```python
from build123d import *

# Parameters (mm, degrees)
SKETCH3_R               = 0.75
CUT_EXTRUDE1_DEPTH      = 1.009552721
CUT_EXTRUDE1_DEPTH_BACK = 5
SKETCH5_R               = 0.830043706
CUT_EXTRUDE3_DEPTH      = 5
SKETCH6_W               = 0.475158235
SKETCH6_H               = 2.253950387
SKETCH6_W_2             = 0.475158234
CUT_EXTRUDE4_DEPTH      = 10
CUT_EXTRUDE4_DEPTH_BACK = 10


with BuildPart() as part:
    # Sketch1 → Revolve1 (revolve)
    with BuildSketch(Plane.XY):
        with BuildLine():
            Line((0, 0), (1, 0))
            Line((1, 0), (1, -12))
            Line((1, -12), (1, -12.602750297))
            add(Edge.make_bspline(
                [(1, -12.602750297), (0.79843866, -14.189468734), (4.052548494, -14.158592974), (3.356440043, -16.677675858), (3.45632985, -17.31657115)],
                knots=[0, 0, 0, 0, 0.610593848, 1, 1, 1, 1], degree=3))
            Line((3.45632985, -17.31657115), (3.084044258, -17.31657115))
            add(Edge.make_bspline(
                [(0, -12.602750297), (-0.217127131, -15.249179965), (3.341761348, -14.727809166), (3.084044258, -17.31657115)],
                knots=[0, 0, 0, 0, 1, 1, 1, 1], degree=3))
            add(Edge.make_bspline(
                [(0, -12), (0, -12.602750297)],
                knots=[0, 0, 1, 1], degree=1))
            Line((0, -12), (0, 0))
        make_face()
    revolve(axis=Axis((3.879111396, 0, 0), (0, -1, 0)))

    # Sketch3 → Cut-Extrude1 (cut, two sides)
    with BuildSketch(Plane(origin=(7.7582228, 0, 0), x_dir=(0, 0, -1), z_dir=(1, 0, 0))) as cut_extrude1_sk:
        with Locations((0, -1.4)):
            Circle(SKETCH3_R)
    extrude(amount=CUT_EXTRUDE1_DEPTH, mode=Mode.SUBTRACT)
    extrude(cut_extrude1_sk.sketch, amount=-CUT_EXTRUDE1_DEPTH_BACK, mode=Mode.SUBTRACT)

    # Sketch5 → Cut-Extrude3 (cut)
    with BuildSketch(Plane(origin=(-0.0208886, 0, 0), x_dir=(0, 0, -1), z_dir=(1, 0, 0))):
        with Locations((0, -1.4)):
            Circle(SKETCH5_R)
    extrude(amount=CUT_EXTRUDE3_DEPTH, mode=Mode.SUBTRACT)

    # Sketch6 → Cut-Extrude4 (cut, two sides)
    with BuildSketch(Plane.XY) as cut_extrude4_sk:
        with Locations((0.237579118, -1.525266711)):
            Rectangle(SKETCH6_W, SKETCH6_H)
        with Locations((7.520643674, -1.525266711)):
            Rectangle(SKETCH6_W_2, SKETCH6_H)
    extrude(amount=CUT_EXTRUDE4_DEPTH, mode=Mode.SUBTRACT)
    extrude(cut_extrude4_sk.sketch, amount=-CUT_EXTRUDE4_DEPTH_BACK, mode=Mode.SUBTRACT)


solid = part.part
```
The listing builds one solid part. Answer for the finished solid, in the listing's coordinates (mm). A direction names the side the tool comes from. Give positions to 0.01 mm unless a question says otherwise; leave off trailing zeros. Order: outer loops, then holes, each group sorted by start corner. A loop starts at its lowest first (then second) coordinate and runs counter-clockwise, first axis right, second up. Notation, with made-up numbers: (-14, 61) - (15, 61) arc R25 ccw to (15, 78) - close; hole circle Ø10 at (-36.5, 13). An arc over 180 degrees is marked (long way). Use one line per item in the form item = value. Start each with the question number.
(1) A cutting plane is placed at A-A, the plane y = -1.4. Write down the section's boundary in (x, z).
(2) The mould has two halves that part along Z. Classify faces 4 (the flat face through (7.283, -2, -1)), 5 (the cylindrical face through (7.754, -6.39, -0.171)), 6 (the cylindrical face through (1.13, -6.39, -0.86)), 7 (the cylindrical face through (6.975, -2.065, -0.346)): released by +Z, released by -Z, zero draft, split by the parting line, or undercut.
(3) A cutting plane is placed at C-C, the plane y = -10.25. Write down the section's boundary in (x, z), then the cut area to 3 significant figures.
(4) A cutting plane is placed at B-B, the plane z = 0. State how many separate pieces and enclosed holes the cut face has, then the cut area to 3 significant figures.
(5) Flat-ended cylindrical pins translate along their axes: pin 1 Ø1.8 at (y, z) = (-1.5, 0) entering from +X; pin 2 Ø2.5 at (y, z) = (-1, 1) entering from -X; pin 3 Ø2 at (x, z) = (1.5, 3) entering from -Y; pin 4 Ø1.3 at (y, z) = (-1.4, 0) entering from -X. Find the tip coordinate at first contact, or state that the pin passes through.
(6) For faces 1 (the flat face through (7, 0, 0)), 2 (the flat face through (0.475, -2, 1)), 3 (the cylindrical face through (0.794, -1.718, -0.767)), determine the directions among +Z, -Z, +X, -X, +Y, -Y from which every point of the face is accessible in a straight line to the end or side of a thin tool.
(7) Consider line 1 (X direction, y = -4.75, z = 0); line 2 (Z direction, x = 3.75, y = -6.75); line 3 (X direction, y = -11, z = -0.5). Determine where each line is inside the solid, lowest interval first. Write a range as from..to.
Ans:
q1.outline = (0.48, -1.86) arc R3.88 ccw to (7.28, -1.86) - (7.28, -0.75) - (6.66, -0.75) arc R2.88 cw to (1.12, -0.83) - (0.48, -0.83) - close; (0.48, 0.83) - (1.12, 0.83) arc R2.88 cw to (6.66, 0.75) - (7.28, 0.75) - (7.28, 1.86) arc R3.88 ccw to (0.48, 1.86) - close
q2.face_4 = zero draft
q2.face_5 = split by the parting line
q2.face_6 = undercut
q2.face_7 = undercut
q3.outline = circle Ø7.76 at (3.88, 0); hole circle Ø5.76 at (3.88, 0)
q3.area = 21.2 mm^2
q4.separate_pieces = 4
q4.enclosed_holes = 0
q4.area = 31.2 mm^2
q5.pin_1 = 7.28
q5.pin_2 = 0
q5.pin_3 = -14.65
q5.pin_4 = through
q6.face_1 = +Z, -Z, +X, -X, +Y
q6.face_2 = +Z, -Z, -X
q6.face_3 = -X
q7.line_1 = 0..1, 6.76..7.76
q7.line_2 = -3.88..-2.88, 2.88..3.88
q7.line_3 = 0.03..1.04, 6.71..7.73
